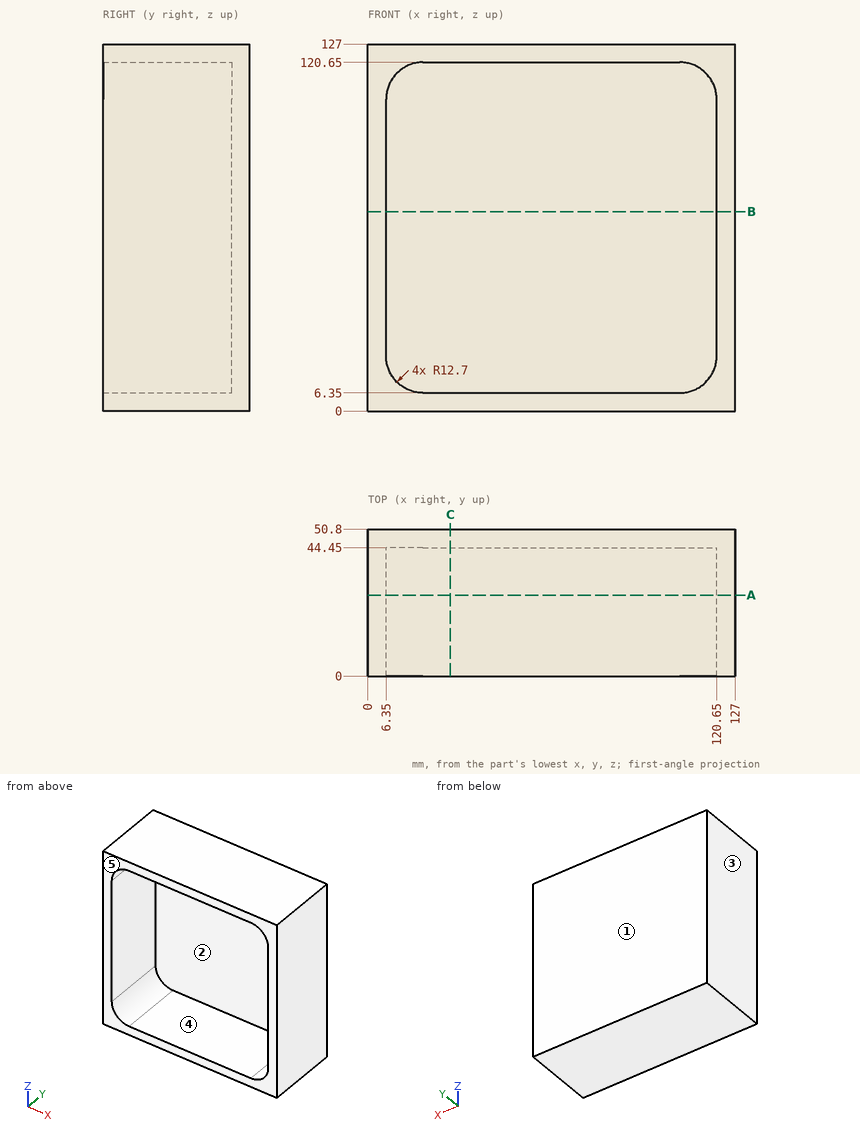
Print and shaded views of the part. All mm, measured from the part's lowest x, y and z. A direction names the side the tool comes from. Coordinates: 2 decimals unless noted, no trailing zeros. Order: outer loops, then holes, each group sorted by start corner. A loop starts at its lowest first (then second) coordinate and runs counter-clockwise, first axis right, second up. Notation, with made-up numbers: (88.25, 82) - (116.25, 82) arc R23 ccw to (116.25, 102) - close; hole circle Ø3 at (71, -21.75). An arc over 180 degrees is marked (long way). Return JSON: item names as keys, results as strings. Group by question number.
Item 1: Cut at A-A (y = 28). List the corners of the cut face in (x, z).
Item 2: Pin check, flat tip, straight feed: pin 1 (4 mm diameter, centred on x = 113.5, z = 92.5, fed in from -Y). Stop position of the tip, or through.
Item 3: Cut at C-C (x = 28.5). List the corners of the cut face in (y, z), plus the area to 3 significant figures.
Item 4: Cut at B-B (z = 69). List the corners of the cut face in (x, y), plus the area to 3 significant figures.
Item 5: Pull direction X, two halves, no side cores. Call the marked faces 1, 2 and 3: pulls with the +X half, pulls with the -X half, needs draft (parallel to the pull), parting line crosses it, or undercut.
Item 6: Which spindle directions (+Z, -Z, +X, -X, +Y, -Y) get a long thin tool onto all of the face, cutting with end or side? Do the marked faces 4 and 5. Say none if no direction does.
Item 7: Drill centre lines: probe 1 along X at (y, z) = (23, 74.5); probe 2 along Y at (x, z) = (25, 17). Where is each one in solid material? Low to high. Write a range as from..to.
Check values:
{
 "1": {"outline": "(0, 0) - (127, 0) - (127, 127) - (0, 127) - close; hole (6.35, 19.05) arc R12.7 ccw to (19.05, 6.35) - (107.95, 6.35) arc R12.7 ccw to (120.65, 19.05) - (120.65, 107.95) arc R12.7 ccw to (107.95, 120.65) - (19.05, 120.65) arc R12.7 ccw to (6.35, 107.95) - close"},
 "2": {"pin 1": "stops at y = 44.45"},
 "3": {"outline": "(0, 0) - (50.8, 0) - (50.8, 127) - (0, 127) - (0, 120.65) - (44.45, 120.65) - (44.45, 6.35) - (0, 6.35) - close", "area": "1,370 mm2"},
 "4": {"outline": "(0, 0) - (6.35, 0) - (6.35, 44.45) - (120.65, 44.45) - (120.65, 0) - (127, 0) - (127, 50.8) - (0, 50.8) - close", "area": "1,370 mm2"},
 "5": {"face 1": "needs draft", "face 2": "undercut", "face 3": "pulls with the -X half"},
 "6": {"face 4": "-Y", "face 5": "+Z, -Z, +X, -X, -Y"},
 "7": {"probe 1": "x = 0..6.35, 120.65..127", "probe 2": "y = 44.45..50.8"}
}
